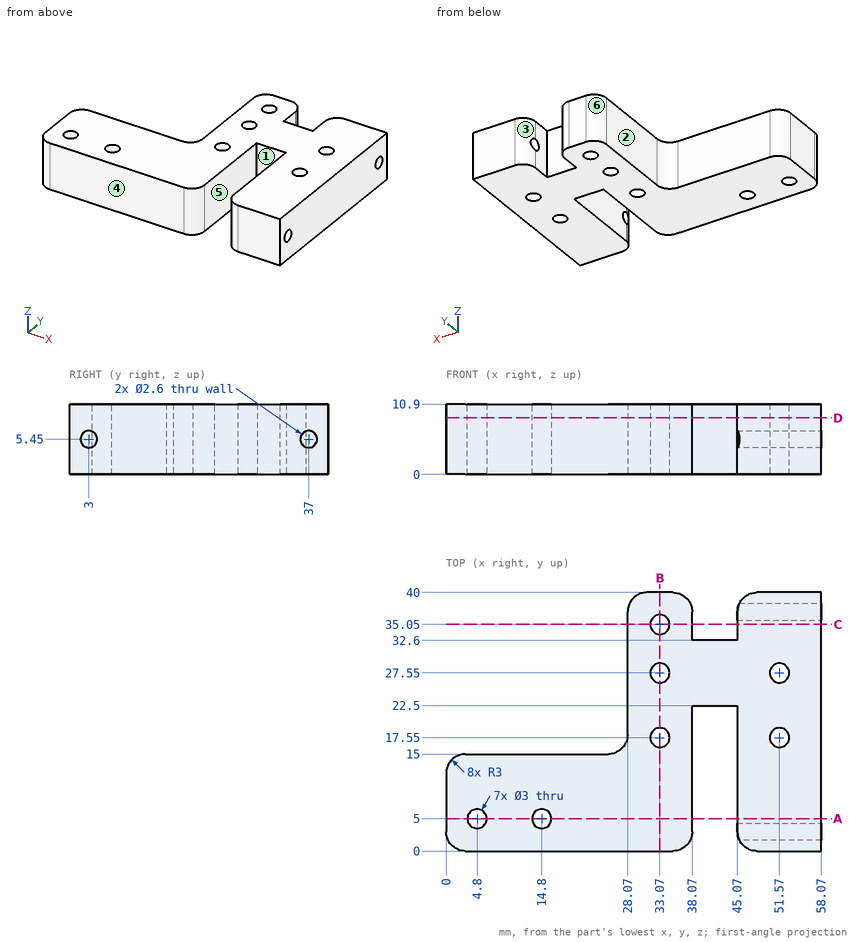
The figure shows three views and two pictorial views of one solid part (mm, origin at its lowest corner). Answer the questions. A direction names the side the tool comes from. Coordinates: 2 decimals unless noted, no trailing zeros. Write each loop counter-clockwise with the first axis right and the second up, starting at its lowest first coordinate (ties: lowest second). Pieces come first, ordered by that corner, then holes.
1. For a pull along X with two mould halves and no side action, classify the marked faces 4, 5 and 6 as +X half, -X half, draft (parallel to the pull), parting line (faces both ways), or undercut.
Results list:
face 4: draft
face 5: undercut
face 6: -X half
2. The part is cut by section D-D, the plane z = 8.75. State how many separate pieces and enclosed holes the cut face has, and give its area (3 significant figures).
Results list:
separate pieces: 1
enclosed holes: 7
area: 1,350 mm2
3. The part is cut by section B-B, the plane x = 33.07. Write down the section's boundary in (y, z).
Results list:
outline: (0, 0) - (16.05, 0) - (16.05, 10.9) - (0, 10.9) - close; (19.05, 0) - (26.05, 0) - (26.05, 10.9) - (19.05, 10.9) - close; (29.05, 0) - (33.55, 0) - (33.55, 10.9) - (29.05, 10.9) - close; (36.55, 0) - (40, 0) - (40, 10.9) - (36.55, 10.9) - close
4. The part is cut by section A-A, the plane y = 5. Write down the section's boundary in (x, z), and give its area (3 significant figures).
Results list:
outline: (0, 0) - (3.3, 0) - (3.3, 10.9) - (0, 10.9) - close; (6.3, 0) - (13.3, 0) - (13.3, 10.9) - (6.3, 10.9) - close; (16.3, 0) - (38.07, 0) - (38.07, 10.9) - (16.3, 10.9) - close; (45.07, 0) - (58.07, 0) - (58.07, 10.9) - (45.07, 10.9) - close
area: 491 mm2
5. Flat-ended cylindrical pins translate along their axes: pin 1 (2 mm diameter, centred on x = 29.5, z = 9, fed in from +Y); pin 2 (4 mm diameter, centred on x = 33.07, y = 35.05, fed in from -Z); pin 3 (6 mm diameter, centred on y = 33, z = 3.5, fed in from -X); pin 4 (1 mm diameter, centred on x = 19.5, z = 9.5, fed in from +Y). Find the tip coordinate at first contact, or state that the pin passes through.
Results list:
pin 1: stops at y = 39.95
pin 2: stops at z = 0
pin 3: stops at x = 28.07
pin 4: stops at y = 15
6. For the marked faces 1, 2 and 3, determine the directions among +Z, -Z, +X, -X, +Y, -Y from which every point of the face is accessible in a straight line to the end or side of a thin tool.
Results list:
face 1: +Z, -Z, -Y
face 2: +Z, -Z, -X, +Y
face 3: +Z, -Z, +Y
7. Consider line 1 along Y through (x, z) = (33.07, 3.25); line 2 along X through (y, z) = (9, 8.5); line 3 along X through (y, z) = (27.5, 1.5). Determine where each line is inside the solid, lowest interval first.
Results list:
line 1: y = 0 to 16.05, 19.05 to 26.05, 29.05 to 33.55, 36.55 to 40
line 2: x = 0 to 38.07, 45.07 to 58.07
line 3: x = 28.07 to 31.57, 34.57 to 50.07, 53.07 to 58.07
8. The part is cut by section C-C, the plane y = 35.05. Write down the section's boundary in (x, z), and give its area (3 significant figures).
Results list:
outline: (28.07, 0) - (31.57, 0) - (31.57, 10.9) - (28.07, 10.9) - close; (34.57, 0) - (38.07, 0) - (38.07, 10.9) - (34.57, 10.9) - close; (45.07, 0) - (58.07, 0) - (58.07, 10.9) - (45.07, 10.9) - close
area: 218 mm2
